```python
from build123d import *

# Parameters (mm, degrees)
BOSS_EXTRUDE1_DEPTH      = 1.75
BOSS_EXTRUDE1_DEPTH_BACK = 14.75
SKETCH1_R                = 3.25
FILLET1_R                = 1.75
SKETCH7_R                = 1.5
CUT_EXTRUDE2_DEPTH       = 0.05
SKETCH1_4_R              = 3.25
SKETCH1_4_R_2            = 2
CUT_EXTRUDE3_DEPTH       = 13
FILLET2_R                = 1.75
CUT_EXTRUDE4_START       = -0.05
SKETCH8_R                = 1.5
CUT_EXTRUDE4_DEPTH       = 0.05


with BuildPart() as part:
    # Sketch1 → Boss-Extrude1 (new, two sides: drawn at the far end of the back side and taken through both)
    with BuildSketch(Plane(origin=(0, 0, 0), x_dir=(1, 0, 0), z_dir=(0, 1, 0)).offset(-BOSS_EXTRUDE1_DEPTH_BACK)):
        with Locations(Location((0, 0, 0), (0, 0, 270))):
            Circle(SKETCH1_R)
        Polygon((0, 1.443375673), (-1.25, 0.721687836), (-1.25, -0.721687836), (0, -1.443375673), (1.25, -0.721687836), (1.25, 0.721687836), align=None, mode=Mode.SUBTRACT)
    extrude(amount=BOSS_EXTRUDE1_DEPTH + BOSS_EXTRUDE1_DEPTH_BACK)

    # Fillet1
    fillet1_edges = [part.edges().sort_by_distance(p)[0] for p in [
        (0, 1.75, -3.25),
    ]]
    fillet(fillet1_edges, radius=FILLET1_R - 0.0001)  # a hair under: the kernel refuses the full size

    # Sketch7 → Cut-Extrude2 (cut)
    with BuildSketch(Plane(origin=(0, 1.75, 0), x_dir=(1, 0, 0), z_dir=(0, 1, 0))):
        with Locations(Location((0, 0, 0), (0, 0, 270))):
            Circle(SKETCH7_R)
    extrude(amount=-CUT_EXTRUDE2_DEPTH, mode=Mode.SUBTRACT)

    # Sketch1<4> → Cut-Extrude3 (cut)
    with BuildSketch(Plane(origin=(0, 0, 0), x_dir=(1, 0, 0), z_dir=(0, 1, 0))):
        with Locations(Location((0, 0, 0), (0, 0, 270))):
            Circle(SKETCH1_4_R)
        with Locations(Location((0, 0, 0), (0, 0, 270))):
            Circle(SKETCH1_4_R_2, mode=Mode.SUBTRACT)
    extrude(amount=-CUT_EXTRUDE3_DEPTH, mode=Mode.SUBTRACT)

    # Fillet2
    fillet2_edges = [part.edges().sort_by_distance(p)[0] for p in [
        (0, -14.75, -3.25),
    ]]
    fillet(fillet2_edges, radius=FILLET2_R - 0.0001)  # a hair under: the kernel refuses the full size

    # Sketch8 → Cut-Extrude4 (cut)
    with BuildSketch(Plane.XZ.offset(14.75).offset(CUT_EXTRUDE4_START)):
        with Locations(Location((0, 0, 0), (0, 0, 90))):
            Circle(SKETCH8_R)
    extrude(amount=CUT_EXTRUDE4_DEPTH, mode=Mode.SUBTRACT)


solid = part.part
```
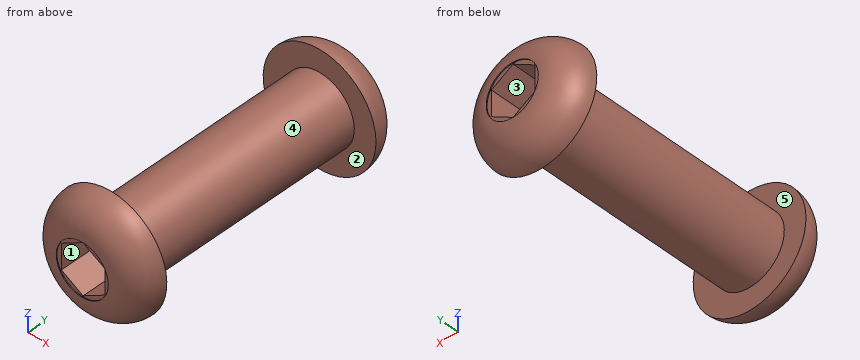
Geometry check sheet. Reference: the model listing, model coordinates, mm. Face numbers are marked on the shaded views. A direction names the side the tool comes from. Coordinates: 2 decimals unless noted, no trailing zeros. Order: outer loops, then holes, each group sorted by start corner. A loop starts at its lowest first (then second) coordinate and runs counter-clockwise, first axis right, second up.
Item 1: Tool access check on the marked faces 1 and 2. Record the directions out of +Z, -Z, +X, -X, +Y, -Y that give a thin tool (end or side, any length) a straight path to the whole face; none if there is none.
Item 2: Scan lines: line 1 along X through (y, z) = (-3.75, 0); line 2 along Z through (x, y) = (1, -8.75); line 3 along Y through (x, z) = (1.25, -2.5). Record each from-to range of solid material in increasing order.
Item 3: Mould release check, pull along Z, two halves, no side actions. Record for the marked faces 3, 4 and 5: released by +Z, released by -Z, zero draft, split by the parting line, or undercut.
Item 4: Depth check by flat-ended pin: pin 1 (3.5 mm diameter, centred on x = 0, z = 0, fed in from +Y); pin 2 (1.5 mm diameter, centred on x = 0.5, z = -0.5, fed in from -Y); pin 3 (1.2 mm diameter, centred on y = -5.5, z = 0, fed in from +X); pin 4 (1 mm diameter, centred on x = -1.5, z = -2.5, fed in from +Y). Enter the tip coordinate at first touch or a pass-through.
Item 5: Section check A-A (y = -5.75). Enter the section's corners in (x, z).
Check sheet entries:
1. face 1: +Y, -Y
1. face 2: none
2. line 1: x = -2 to -1.25, 1.25 to 2
2. line 2: z = -1.73 to -0.87, 0.87 to 1.73
2. line 3: y = -14.18 to -13, 0 to 1.18
3. face 3: undercut
3. face 4: split by the parting line
3. face 5: zero draft
4. pin 1: stops at y = 1.75
4. pin 2: stops at y = -14.7
4. pin 3: stops at x = 2
4. pin 4: stops at y = 1.49
5. outline: circle Ø4 at (0, 0); hole (-1.25, -0.72) - (0, -1.44) - (1.25, -0.72) - (1.25, 0.72) - (0, 1.44) - (-1.25, 0.72) - close
